Could you check a few things on this model? Use its own coordinates, in mm. A direction names the side the tool comes from. Coordinates: 2 decimals unless noted, no trailing zeros. Order: outer loops, then holes, each group sorted by start corner. A loop starts at its lowest first (then second) coordinate and runs counter-clockwise, first axis right, second up. Notation, with made-up numbers: (-23, 41) - (-9, 41) arc R20 cw to (-9, 70) - close; hole circle Ø8 at (12.25, -19.5). An arc over 180 degrees is marked (long way). One line per item, written item: value. Start each with the question number.
from build123d import *
from build123d.topology import SkipClean

# Parameters (mm, degrees)
SKETCH1_R           = 30
BOSS_EXTRUDE1_DEPTH = 25
FILLET1_R           = 3
SKETCH3_R           = 22.5
CUT_EXTRUDE1_DEPTH  = 20
CHAMFER1_SIZE       = 3
CUT_EXTRUDE2_DEPTH  = 50.244289131
CIRPATTERN1_COUNT   = 5
CIRPATTERN1_ANGLE   = 284
SKETCH4_R           = 10
BOSS_EXTRUDE2_DEPTH = 15
SKETCH5_R           = 3
CUT_EXTRUDE3_DEPTH  = 47.904157726
SKETCH6_R           = 2
CUT_EXTRUDE4_DEPTH  = 50.244289131
SKETCH7_R           = 4
CUT_EXTRUDE5_DEPTH  = 64.442887868


with BuildPart() as part:
    # Sketch1 → Boss-Extrude1 (new body)
    with BuildSketch(Plane(origin=(0, 0, 0), x_dir=(0, 0, -1), z_dir=(1, 0, 0))):
        Circle(SKETCH1_R)
    extrude(amount=BOSS_EXTRUDE1_DEPTH)

    # Fillet1
    fillet1_edges = [part.edges().sort_by_distance(p)[0] for p in [
        (0, 0, 30),
        (25, 0, 30),
    ]]
    fillet(fillet1_edges, radius=FILLET1_R)

    # Sketch3 → Cut-Extrude1 (cut)
    with BuildSketch(Plane.ZY):
        Circle(SKETCH3_R)
    extrude(amount=-CUT_EXTRUDE1_DEPTH, mode=Mode.SUBTRACT)

    # Chamfer1
    chamfer1_edges = [part.edges().sort_by_distance(p)[0] for p in [
        (0, 0, -22.5),
    ]]
    chamfer(chamfer1_edges, length=CHAMFER1_SIZE)

    # Sketch2 → Cut-Extrude2 (cut, through all)
    with BuildSketch(Plane.ZY.offset(-25)):
        with BuildLine():
            Line((-6.233158363, 10.835023619), (-11.219685054, 19.503042514))
            ThreePointArc((-11.219685054, 19.503042514), (-15.885142396, 15.934624283), (-19.468053536, 11.280287741))
            Line((-19.468053536, 11.280287741), (-10.815585298, 6.266826523))
            ThreePointArc((-10.815585298, 6.266826523), (-8.825079109, 8.852569046), (-6.233158363, 10.835023619))
        make_face()
    cut_extrude2 = extrude(amount=CUT_EXTRUDE2_DEPTH, mode=Mode.SUBTRACT)

    # CirPattern1: Cut-Extrude2 ×5 about axis
    with SkipClean():  # the faces are left unmerged after this step: merging them gives an invalid solid
        cirpattern1_axis = Axis((0, 0, 0), (1, 0, 0))
        for i in range(1, CIRPATTERN1_COUNT):
            add(cut_extrude2.rotate(cirpattern1_axis, i * CIRPATTERN1_ANGLE / (CIRPATTERN1_COUNT - 1)), mode=Mode.SUBTRACT)
    add(part.part.scale(1), mode=Mode.REPLACE)  # the faces are merged on a copy

    # Sketch4 → Boss-Extrude2 (add)
    with BuildSketch(Plane.ZY.offset(-20)):
        Circle(SKETCH4_R)
    extrude(amount=BOSS_EXTRUDE2_DEPTH)

    # Sketch5 → Cut-Extrude3 (cut, through all)
    with BuildSketch(Plane.ZY.offset(-5)):
        Circle(SKETCH5_R)
    extrude(amount=-CUT_EXTRUDE3_DEPTH, mode=Mode.SUBTRACT)

    # Sketch6 → Cut-Extrude4 (cut, through all)
    with BuildSketch(Plane(origin=(0, 0, 0), x_dir=(1, 0, 0), z_dir=(0, 1, 0))):
        with Locations(Location((12.5, 0, 0), (0, 0, 270))):
            Circle(SKETCH6_R)
    extrude(amount=-CUT_EXTRUDE4_DEPTH, mode=Mode.SUBTRACT)

    # Sketch7 → Cut-Extrude5 (cut, through all)
    with BuildSketch(Plane(origin=(0, -20, 0), x_dir=(1, 0, 0), z_dir=(0, 1, 0))):
        with Locations(Location((12.5, 0, 0), (0, 0, 270))):
            Circle(SKETCH7_R)
    extrude(amount=-CUT_EXTRUDE5_DEPTH, mode=Mode.SUBTRACT)


solid = part.part
Q1. I want a section at D-D on y = 15. State how many separate pieces and enclosed holes the cut face has, then the cut area to 3 significant figures.
Q2. I'm going to push flat-ended pins straight in: pin 1 (2 mm diameter, centred on x = 14.5, z = -5, fed in from -Y); pin 2 (5 mm diameter, centred on x = 5.5, y = -3, fed in from -Z); pin 3 (12 mm diameter, centred on x = 5, y = 9, fed in from -Z); pin 4 (9 mm diameter, centred on x = 12.5, z = 0, fed in from -Y). Where does each tip first touch, or does it pass through?
Q3. If I drill on L1, parallel to Y at x = 18.75, z = 0; L2, parallel to Y at x = 20.5, z = 0; L3, parallel to X at y = -27, z = 0, over which ranges is the centre line in solid material (lowest first)?
Q4. I want a section at B-B on x = 4.25. Please give me the cut outline in (y, z), then the cut area to 3 significant figures.
Q5. I want a section at A-A on x = 12.5. Please give me the cut outline in (y, z).
Q6. Which directions (+Z, -Z, +X, -X, +Y, -Y) give clear straight access to the entire face, cutting with the end or side of a thin tool? Please do faces 1 (the cylindrical face through (12.6, -9.76, -2.17)), 2 (the flat face through (22.535, -15.667, 7.952)), 3 (the cylindrical face through (12.588, -6.066, -1.998)).
Q7. I want a section at C-C on x = 23.25. Please give me the cut outline in (y, z), then the cut area to 3 significant figures.
Q8. We'd pull the mould along X, two halves only. Please class faces 4 (the flat face through (20, 10.3, -0.4)), 5 (the cylindrical face through (16.466, -26.02, -0.521)), 6 (the flat face through (22.535, 2.418, 17.403)), 7 (the flat face through (25, -6, 0)): +X half, -X half, draft (parallel to the pull), parting line (faces both ways), or undercut.
Values follow:
1. separate pieces: 3
1. enclosed holes: 0
1. area: 516 mm^2
2. pin 1: stops at y = -29.73
2. pin 2: stops at z = -30
2. pin 3: stops at z = -29.85
2. pin 4: stops at y = -30
3. L1: y = -30 to -22.5, -10 to -3, 3 to 10, 22.5 to 30
3. L2: y = -30 to -22.5, -12.5 to -3, 3 to 30
3. L3: x = 0 to 8.5, 16.5 to 25
4. outline: circle Ø60 at (0, 0); hole circle Ø45 at (0, 0)
4. area: 1,240 mm^2
5. outline: (-29.73, -4) arc R30 ccw (long way) to (-29.73, 4) - (-22.14, 4) arc R22.5 cw (long way) to (-22.14, -4) - close; (-9.8, -2) arc R10 ccw (long way) to (-9.8, 2) - (-2.24, 2) arc R3 cw (long way) to (-2.24, -2) - close
6. face 1: -X
6. face 2: +X, -X
6. face 3: -Y
7. outline: circle Ø59.45 at (0, 0); hole (-22.47, -1.21) - (-12.48, -0.67) arc R12.5 cw to (-11.15, 5.66) - (-20.06, 10.18) arc R22.5 ccw to start; hole (-16.16, -15.65) arc R22.5 ccw to (-6.17, -21.64) - (-3.43, -12.02) arc R12.5 cw to (-8.98, -8.7) - close; hole (-8.46, 20.85) - (-4.7, 11.58) arc R12.5 cw to (1.72, 12.38) - (3.1, 22.29) arc R22.5 ccw to start; hole circle Ø6 at (0, 0); hole (6.27, -10.82) - (11.28, -19.47) arc R22.5 ccw to (19.5, -11.22) - (10.84, -6.23) arc R12.5 cw to start; hole (9.42, 8.22) arc R12.5 cw to (12.27, 2.4) - (22.08, 4.33) arc R22.5 ccw to (16.96, 14.79) - close
7. area: 2,290 mm^2
8. face 4: -X half
8. face 5: undercut
8. face 6: draft
8. face 7: +X half
